from build123d import *

# Parameters (mm, degrees)
SKETCH5_R           = 4
BOSS_EXTRUDE2_DEPTH = 4
BOSS_EXTRUDE3_DEPTH = 4
SKETCH7_R           = 2.6
CUT_EXTRUDE3_DEPTH  = 2.5
BOSS_EXTRUDE4_DEPTH = 2.5
FILLET1_R           = 0.3
SKETCH9_W           = 4
SKETCH9_H           = 10
BOSS_EXTRUDE5_DEPTH = 7
CUT_EXTRUDE4_REACH  = 29.603
CHAMFER1_SIZE       = 16
CHAMFER1_SIZE2      = 5.823523748
CHAMFER2_SIZE       = 7
CHAMFER2_SIZE2      = 2.54779164
FILLET5_R           = 5
FILLET6_R           = 12
FILLET7_R           = 2


with BuildPart() as part:
    # Sketch5 → Boss-Extrude2 (new body)
    with BuildSketch(Plane(origin=(0, 0, 0), x_dir=(0, 0, -1), z_dir=(1, 0, 0))):
        Circle(SKETCH5_R)
    extrude(amount=BOSS_EXTRUDE2_DEPTH)

    # Sketch6 → Boss-Extrude3 (add)
    with BuildSketch(Plane(origin=(0, 0, 0), x_dir=(0, 0, -1), z_dir=(1, 0, 0))):
        Polygon((-2.571150439, 3.064177772), (2.571150439, -3.064177772), (-12.366716202, -15.598536161), (-17.50901708, -9.470180616), align=None)
    extrude(amount=BOSS_EXTRUDE3_DEPTH)

    # Sketch7 → Cut-Extrude3 (cut)
    with BuildSketch(Plane.ZY):
        Circle(SKETCH7_R)
    extrude(amount=-CUT_EXTRUDE3_DEPTH, mode=Mode.SUBTRACT)

    # Sketch8 → Boss-Extrude4 (add)
    with BuildSketch(Plane.ZY.offset(-2.5)):
        Polygon((1.6, -0.75), (-1.6, -0.75), (-1.6, 0.75), (-0.65, 0.75), (-0.65, 1.25), (0.65, 1.25), (0.65, 0.75), (1.6, 0.75), align=None)
    extrude(amount=BOSS_EXTRUDE4_DEPTH)

    # Fillet1
    fillet1_edges = [part.edges().sort_by_distance(p)[0] for p in [
        (1.25, -0.75, 1.6),
        (1.25, 0.75, 1.6),
        (1.25, 0.75, -1.6),
        (1.25, -0.75, -1.6),
    ]]
    fillet(fillet1_edges, radius=FILLET1_R)

    # Sketch9 → Boss-Extrude5 (add)
    with BuildSketch(Plane(origin=(0, -3.064177772, -2.571150439), x_dir=(1, 0, 0), z_dir=(0, -0.766044443118976, -0.6427876096865419))):
        with Locations((2, 14.5)):
            Rectangle(SKETCH9_W, SKETCH9_H)
    extrude(amount=BOSS_EXTRUDE5_DEPTH)

    # Sketch10 → Cut-Extrude4 (cut, up to next)
    with BuildSketch(Plane(origin=(4, 0, 0), x_dir=(0, 0, -1), z_dir=(1, 0, 0)), mode=Mode.PRIVATE) as cut_extrude4_sk1:
        with BuildLine():
            Line((-4.00251634, -13.097436491), (-6.50251634, -17.427563509))
            ThreePointArc((-6.50251634, -17.427563509), (-8.3125, -17.912547169), (-8.79748366, -16.102563509))
            Line((-8.79748366, -16.102563509), (-6.29748366, -11.772436491))
            ThreePointArc((-6.29748366, -11.772436491), (-4.4875, -11.287452831), (-4.00251634, -13.097436491))
        make_face()
    cut_extrude4_tool1 = extrude(cut_extrude4_sk1.sketch, amount=-CUT_EXTRUDE4_REACH, mode=Mode.PRIVATE) & part.part
    add(cut_extrude4_tool1.solids().sort_by_distance((4, -14.6, 6.4))[0], mode=Mode.SUBTRACT)

    # Chamfer1
    chamfer1_edges = [part.edges().sort_by_distance(p)[0] for p in [
        (2, -9.470180616, 17.50901708),
    ]]
    chamfer1_side = [part.faces().sort_by_distance(p)[0] for p in [
        (2, -3.203001422, 10.040083759),
    ]]
    chamfer(chamfer1_edges, length=CHAMFER1_SIZE, length2=CHAMFER1_SIZE2, reference=chamfer1_side[0])

    # Chamfer2
    chamfer2_edges = [part.edges().sort_by_distance(p)[0] for p in [
        (2, -14.532971166, 0.206758503),
    ]]
    chamfer2_side = [part.faces().sort_by_distance(p)[0] for p in [
        (2, -17.746909215, 4.036980719),
    ]]
    chamfer(chamfer2_edges, length=CHAMFER2_SIZE, length2=CHAMFER2_SIZE2, reference=chamfer2_side[0])

    # Fillet5
    # the kernel refuses this fillet: 5 mm, written as the material it adds along each edge
    with BuildSketch(Plane(origin=(4, -9.170660064, 4.706271771), x_dir=(0, -0.7660444431189757, -0.6427876096865421), z_dir=(-1, 0, 0))) as fillet5_piece_1:
        with BuildLine():
            CenterArc((5, -4.969901842), FILLET5_R, 96.289855747, 83.710144253)
            Line((0, -4.969901842), (-0.1, -4.969901842))
            Line((-0.1, -4.969901842), (-0.1, 0))
            Line((-0.1, 0), (0, 0.1))
            ThreePointArc((0, 0.1), (2.22610418, 0.1), (4.441252527, 0.099398037))
            Line((4.441252527, 0.099398037), (4.45220836, 0))
        make_face()
    extrude(amount=4)

    # Fillet6
    fillet6_edges = [part.edges().sort_by_distance(p)[0] for p in [
        (2, -13.931258623, 13.765728169),
    ]]
    fillet(fillet6_edges, radius=FILLET6_R)

    # Fillet7
    fillet7_edges = [part.edges().sort_by_distance(p)[0] for p in [
        (2, -12.581249538, 1.844447401),
        (2, -20.960847263, 7.867202934),
    ]]
    fillet(fillet7_edges, radius=FILLET7_R)


solid = part.part
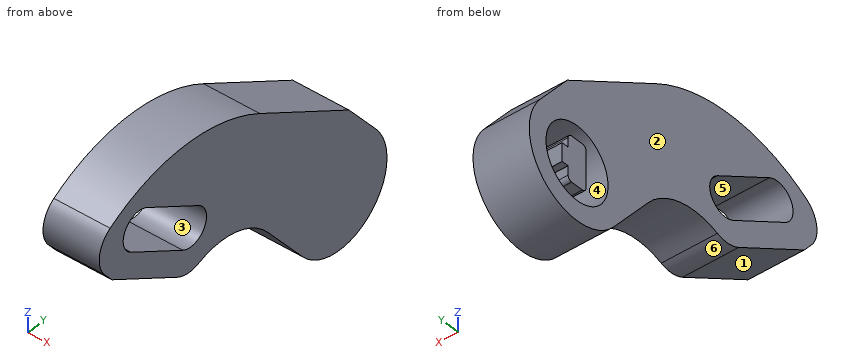
Could you check a few things on this model? Use its own coordinates, in mm. Face numbers are marked on the shaded views. A direction names the side the tool comes from. Give positions to 0.01 mm unless a question says otherwise; leave off trailing zeros. Loops run counter-clockwise (first coordinate to the right, second up) from the corner with the lowest first, then second, coordinate; pieces in that order, holes last. Notation, with made-up numbers: M 21,79 L 45,79 A19 cw 45,84 Z; hole C 7.25,62.5 d2. An arc over 180 degrees is marked long. Answer as a JSON object with one key per item and string values.
Q1. For P1, Ø1.5, axis at x = 1.5, y = -7, coming from the -Z side; P2, Ø1.2, axis at x = 1.5, z = 0, coming from the -Y side; P3, Ø0.5, axis at x = 1, z = 1, coming from the +Y side, each with a flat end and sliding along its axis, tell me the tip position at first contact or that it passes through.
Values found:
{"P1": "stops at z = 1.2", "P2": "stops at y = -5.73", "P3": "stops at y = 3.93"}
Q2. If I drill on probe 1 along Y at (x, z) = (0.6, 0); probe 2 along Y at (x, z) = (2.45, -0.5); probe 3 along Z at (x, y) = (1.35, -0.5), over which ranges is the centre line in solid material (lowest first)? Write a range as [from, to].
Values found:
{"probe 1": "y = [-5.22, -2.6], [-0.75, 1.25], [2.6, 4]", "probe 2": "y = [-4.8, -2.55], [-0.75, 1.25], [2.55, 3.97]", "probe 3": "z = [-3.97, -2.55], [-1.6, 1.6], [2.55, 6.01]"}
Q3. Suppose I cut it at C-C, the plane x = 1.45. State how many separate pieces and enclosed holes the cut face has, plus the area to 3 significant figures.
Values found:
{"separate pieces": "2", "enclosed holes": "2", "area": "152 mm²"}
Q4. If we mould it in two halves opening along Z, with no side actions, what happens to the marked faces 1, 2 and 3? For each: pulls with the +Z half, pulls with the -Z half, needs draft (parallel to the pull), parting line crosses it, or undercut.
Values found:
{"face 1": "pulls with the -Z half", "face 2": "needs draft", "face 3": "undercut"}
Q5. For the marked faces 4, 5 and 6, which set-ups out of +Z, -Z, +X, -X, +Y, -Y let a thin tool reach every point of the face, with its end or its side?
Values found:
{"face 4": "-X", "face 5": "+X, -X", "face 6": "-Z, +X, -X"}
Q6. Suppose I cut it at A-A, the plane z = 4.25. List the corners of the cut face in (x, y) for me.
Values found:
{"outline": "M 0,-16.75 L 4,-16.75 L 4,-13.53 L 0,-13.53 Z; M 0,-11.46 L 4,-11.46 L 4,1.66 L 0,1.66 Z"}
Q7. Suppose I cut it at B-B, the plane y = 0. List the corners of the cut face in (x, z) for me.
Values found:
{"outline": "M 0,-4 L 4,-4 L 4,5.72 L 0,5.72 L 0,2.6 L 2.5,2.6 L 2.5,1.6 L 0,1.6 L 0,-1.6 L 2.5,-1.6 L 2.5,-2.6 L 0,-2.6 Z"}
Q8. Suppose I cut it at D-D, the plane z = 0. List the corners of the cut face in (x, y) for me.
Values found:
{"outline": "M 0,-5.22 L 4,-5.22 L 4,4 L 0,4 L 0,2.6 L 2.5,2.6 L 2.5,1.25 L 0,1.25 L 0,-0.75 L 2.5,-0.75 L 2.5,-2.6 L 0,-2.6 Z"}
